```python
from build123d import *

# Parameters (mm, degrees)
SKETCH_W        = 50
SKETCH_H        = 50
PAD_DEPTH       = 10
SKETCH001_W     = 15
SKETCH001_H     = 50
PAD001_DEPTH    = 140
SKETCH004_R     = 2.6
POCKET002_DEPTH = 10
SKETCH005_R     = 8.5
SKETCH005_R_2   = 2.66237
SKETCH005_R_3   = 2.705532
POCKET_DEPTH    = 15
SKETCH006_W     = 50
SKETCH006_H     = 55
PAD002_DEPTH    = 50
SKETCH009_W     = 8
SKETCH009_H     = 50
PAD003_DEPTH    = 15
SKETCH010_R     = 8.5
POCKET003_DEPTH = 65
SKETCH011_R     = 18.1
POCKET004_DEPTH = 18
SKETCH012_R     = 2.570984
SKETCH012_R_2   = 2.587377
SKETCH012_R_3   = 2.575599
SKETCH012_R_4   = 2.613837
POCKET005_DEPTH = 65
CHAMFER_SIZE    = 7
CHAMFER001_SIZE = 7
SKETCH013_W     = 83.432911
SKETCH013_H     = 55
PAD004_DEPTH    = 4
SKETCH014_W     = 4
SKETCH014_H     = 55
PAD005_DEPTH    = 46
PAD006_DEPTH    = 4
PAD007_DEPTH    = 4
POCKET006_DEPTH = 5
SKETCH018_W     = 40
SKETCH018_H     = 35
PAD008_DEPTH    = 4
SKETCH019_R     = 1.6
POCKET007_DEPTH = 5
PAD009_DEPTH    = 3
PAD010_DEPTH    = 3
SKETCH022_R     = 2.1
POCKET008_DEPTH = 10
PAD011_DEPTH    = 50


with BuildPart() as part:
    # Sketch → Pad (new body)
    with BuildSketch(Plane.XY):
        with Locations((0, 25)):
            Rectangle(SKETCH_W, SKETCH_H)
    extrude(amount=PAD_DEPTH)

    # Sketch001 (on Face6 of Pad) → Pad001 (join)
    with BuildSketch(Plane.XY.offset(10)):
        with Locations((0, 25)):
            Rectangle(SKETCH001_W, SKETCH001_H)
    extrude(amount=PAD001_DEPTH)

    # Sketch004 → Pocket002 (cut)
    with BuildSketch(Plane(origin=(0, 0, 0), x_dir=(1, 0, 0), z_dir=(0, 0, -1))):
        with Locations((-20, -13)):
            Circle(SKETCH004_R)
        with Locations((20, -13)):
            Circle(SKETCH004_R)
        with Locations((-20, -37)):
            Circle(SKETCH004_R)
        with Locations((20, -37)):
            Circle(SKETCH004_R)
    extrude(amount=-POCKET002_DEPTH, mode=Mode.SUBTRACT)

    # Sketch005 (on Face14 of Pocket002) → Pocket (cut)
    with BuildSketch(Plane.YZ.offset(7.5)):
        with Locations((25, 50)):
            Circle(SKETCH005_R)
        with Locations((25, 120)):
            Circle(SKETCH005_R)
        with Locations((39.142136, 64.142136)):
            Circle(SKETCH005_R_2)
        with Locations((10.857864, 35.857864)):
            Circle(SKETCH005_R_3)
    extrude(amount=-POCKET_DEPTH, mode=Mode.SUBTRACT)

    # Sketch006 (on Face13 of Pocket) → Pad002 (join)
    with BuildSketch(Plane(origin=(-7.5, 0, 0), x_dir=(0, -1, 0), z_dir=(-1, 0, 0))):
        with Locations((-25, 122.5)):
            Rectangle(SKETCH006_W, SKETCH006_H)
    extrude(amount=PAD002_DEPTH)

    # Sketch009 → Pad003 (join)
    with BuildSketch(Plane.XY.offset(10)):
        with Locations((11.5, 25)):
            Rectangle(SKETCH009_W, SKETCH009_H)
        with Locations((-11.5, 25)):
            Rectangle(SKETCH009_W, SKETCH009_H)
    extrude(amount=PAD003_DEPTH)

    # Sketch010 (on Face34 of Pad003) → Pocket003 (cut)
    with BuildSketch(Plane.YZ.offset(-7.5)):
        with Locations((25, 120)):
            Circle(SKETCH010_R)
    extrude(amount=-POCKET003_DEPTH, mode=Mode.SUBTRACT)

    # Sketch011 (on DatumPlane) → Pocket004 (cut)
    with BuildSketch(Plane(origin=(-57.5, 0, 0), x_dir=(0, -1, 0), z_dir=(-1, 0, 0))):
        with Locations((-25, 120)):
            Circle(SKETCH011_R)
    extrude(amount=-POCKET004_DEPTH, mode=Mode.SUBTRACT)

    # Sketch012 (on DatumPlane) → Pocket005 (cut)
    with BuildSketch(Plane(origin=(-57.5, 0, 0), x_dir=(0, -1, 0), z_dir=(-1, 0, 0))):
        with Locations((-40.525694, 104.474306)):
            Circle(SKETCH012_R)
        with Locations((-40.524277, 135.524276)):
            Circle(SKETCH012_R_2)
        with Locations((-9.47356, 135.526441)):
            Circle(SKETCH012_R_3)
        with Locations((-9.442338, 104.444964)):
            Circle(SKETCH012_R_4)
    extrude(amount=-POCKET005_DEPTH, mode=Mode.SUBTRACT)

    # Chamfer
    chamfer_edges = [part.edges().sort_by_distance(p)[0] for p in [
        (15.5, 25, 25),
    ]]
    chamfer(chamfer_edges, length=CHAMFER_SIZE)

    # Chamfer001
    chamfer001_edges = [part.edges().sort_by_distance(p)[0] for p in [
        (-15.5, 25, 25),
    ]]
    chamfer(chamfer001_edges, length=CHAMFER001_SIZE)

    # Sketch013 (on DatumPlane) → Pad004 (join)
    with BuildSketch(Plane(origin=(0, 50, 0), x_dir=(-1, 0, 0), z_dir=(0, 1, 0))):
        with Locations((33.993362, 122.5)):
            Rectangle(SKETCH013_W, SKETCH013_H)
    extrude(amount=PAD004_DEPTH)

    # Sketch014 (on Face47 of Pad004) → Pad005 (join)
    with BuildSketch(Plane(origin=(0, 54, 0), x_dir=(-1, 0, 0), z_dir=(0, 1, 0))):
        with Locations((73.710442, 122.5)):
            Rectangle(SKETCH014_W, SKETCH014_H)
    extrude(amount=PAD005_DEPTH)

    # Sketch015 (on DatumPlane) → Pad006 (join)
    with BuildSketch(Plane.XY.offset(150)):
        Polygon((-71.717157, 54), (-11.717157, 54), (-71.717157, 87), align=None)
    extrude(amount=-PAD006_DEPTH)

    # Sketch016 (on DatumPlane) → Pad007 (join)
    with BuildSketch(Plane(origin=(0, 0, 95), x_dir=(1, 0, 0), z_dir=(0, 0, -1))):
        Polygon((-71.768631, -54), (-11.768631, -54), (-71.768631, -87), align=None)
    extrude(amount=-PAD007_DEPTH)

    # Sketch017 (on DatumPlane) → Pocket006 (cut)
    with BuildSketch(Plane(origin=(-75.710442, 0, 0), x_dir=(0, -1, 0), z_dir=(-1, 0, 0))):
        with BuildLine():
            ThreePointArc((-58.500315, 102.966849), (-56.900315, 104.566849), (-58.500315, 106.166849))
            Line((-58.500315, 106.166849), (-65.500315, 106.166849))
            ThreePointArc((-65.500315, 106.166849), (-67.100315, 104.566849), (-65.500315, 102.966849))
            Line((-65.500315, 102.966849), (-58.500315, 102.966849))
        make_face()
        with BuildLine():
            ThreePointArc((-89.5, 103.106524), (-87.9, 104.706524), (-89.5, 106.306524))
            Line((-89.5, 106.306524), (-96.5, 106.306524))
            ThreePointArc((-96.5, 106.306524), (-98.1, 104.706524), (-96.5, 103.106524))
            Line((-96.5, 103.106524), (-89.5, 103.106524))
        make_face()
        with BuildLine():
            ThreePointArc((-89.500832, 133.9), (-87.900832, 135.5), (-89.500832, 137.1))
            Line((-89.500832, 137.1), (-96.500832, 137.1))
            ThreePointArc((-96.500832, 137.1), (-98.100832, 135.5), (-96.500832, 133.9))
            Line((-96.500832, 133.9), (-89.500832, 133.9))
        make_face()
        with BuildLine():
            ThreePointArc((-58.500832, 133.9), (-56.900832, 135.5), (-58.500832, 137.1))
            Line((-58.500832, 137.1), (-65.500832, 137.1))
            ThreePointArc((-65.500832, 137.1), (-67.100832, 135.5), (-65.500832, 133.9))
            Line((-65.500832, 133.9), (-58.500832, 133.9))
        make_face()
        with BuildLine():
            ThreePointArc((-69.87661, 109), (-58.87661, 120), (-69.87661, 131))
            Line((-69.87661, 131), (-83.87661, 131))
            ThreePointArc((-83.87661, 131), (-94.87661, 120), (-83.87661, 109))
            Line((-83.87661, 109), (-69.87661, 109))
        make_face()
    extrude(amount=-POCKET006_DEPTH, mode=Mode.SUBTRACT)

    # Sketch018 (on DatumPlane) → Pad008 (join)
    with BuildSketch(Plane.XY.offset(150)):
        with Locations((-20, -17.5)):
            Rectangle(SKETCH018_W, SKETCH018_H)
    extrude(amount=-PAD008_DEPTH)

    # Sketch019 (on DatumPlane) → Pocket007 (cut)
    with BuildSketch(Plane.XY.offset(150)):
        with Locations((-10, -10)):
            Circle(SKETCH019_R)
        with Locations((-10, -25)):
            Circle(SKETCH019_R)
        with Locations((-35, -10)):
            Circle(SKETCH019_R)
        with Locations((-35, -25)):
            Circle(SKETCH019_R)
    extrude(amount=-POCKET007_DEPTH, mode=Mode.SUBTRACT)

    # Sketch020 (on DatumPlane) → Pad009 (join)
    with BuildSketch(Plane.YZ):
        Polygon((0, 146.040518), (-25, 146.040518), (0, 136.040518), align=None)
    extrude(amount=-PAD009_DEPTH)

    # Sketch021 (on DatumPlane) → Pad010 (join)
    with BuildSketch(Plane(origin=(-40, 0, 0), x_dir=(0, -1, 0), z_dir=(-1, 0, 0))):
        Polygon((0, 146), (25, 146), (0, 136), align=None)
    extrude(amount=-PAD010_DEPTH)

    # Sketch022 (on Face6 of Pocket006) → Pocket008 (cut)
    with BuildSketch(Plane.XZ):
        with Locations((0, 44.95862)):
            Circle(SKETCH022_R)
        with Locations((0, 64.95862)):
            Circle(SKETCH022_R)
    extrude(amount=-POCKET008_DEPTH, mode=Mode.SUBTRACT)

    # Sketch023 (on DatumPlane) → Pad011 (join)
    with BuildSketch(Plane.XZ):
        Polygon((-7.495659, 95), (-7.495659, 75), (-57.495659, 95), align=None)
    extrude(amount=-PAD011_DEPTH)


solid = part.part
```
The model under review builds one solid part; all positions refer to its coordinate system, in mm. A direction names the side the tool comes from. Coordinates: 2 decimals unless noted, no trailing zeros. Write each loop counter-clockwise with the first axis right and the second up, starting at its lowest first coordinate (ties: lowest second). Pieces come first, ordered by that corner, then holes. Notation, with made-up numbers: (-1.75, 68) -> (22.25, 68) arc R36 cw to (22.25, 103) -> close; hole circle Ø9 at (34.5, 38.25). An arc over 180 degrees is marked (long way). One line per item, written item: value. Start each with the question number.
Q1. Clearance check with flat-ended pins moving along their axes: P1, Ø1.3, axis at x = -0.5, z = 44.5, coming from the -Y side; P2, Ø6, axis at y = 24.5, z = 56.5, coming from the -X side; P3, Ø5, axis at x = 0, z = 44.96, coming from the -Y side. State where each tip first meets the part, or that it passes through.
Q2. Add section B-B, the plane x = 20. Give the boundary of the cut face in (y, z), then the cut area to 3 significant figures.
Q3. Add section A-A, the plane z = 120. Count the separate pieces of the cut face and the enclosed holes in it, then the cut area to 3 significant figures.
Q4. The part is to be moulded in two halves that separate along Y. For faces 4 (the face through (21.2, 15.307, 4.93)), 5 (the face through (-49, 65, 95)), 6 (the face through (0, 10, 65)), say which applies: +Y half, -Y half, draft (parallel to the pull), parting line (faces both ways), or undercut.
Q5. To check wall thickness, follow probe 1 along Y at (x, z) = (20, 2.25); probe 2 along Y at (x, z) = (-10, 148.3); probe 3 along Z at (x, y) = (-23, 26.5). State the ranges of each line that lie inside material, in increasing order.
Q6. For faces 1 (the face through (-20, 25, 10)), 2 (the face through (-0.27, 4.93, 67.04)), 3 (the face through (-17, 0, 91)), list the 3-axis set-ups (+Z, -Z, +X, -X, +Y, -Y) from which the entire face can be reached by the end or side of a thin tool; tool diameter is ignored.
Q7. Add section D-D, the plane y = 81. Give the boundary of the cut face in (x, z).
Response:
1. P1: y = 10
1. P2: x = -7.5
1. P3: y = 0
2. outline: (0, 0) -> (10.4, 0) -> (10.4, 10) -> (0, 10) -> close; (15.6, 0) -> (34.4, 0) -> (34.4, 10) -> (15.6, 10) -> close; (39.6, 0) -> (50, 0) -> (50, 10) -> (39.6, 10) -> close
2. area: 396 mm²
3. separate pieces: 3
3. enclosed holes: 0
3. area: 2,170 mm²
4. face 4: undercut
4. face 5: draft
4. face 6: -Y half
5. probe 1: 0 to 10.4, 15.6 to 34.4, 39.6 to 50
5. probe 2: -35 to -26.6, -23.4 to -11.6, -8.4 to 54
5. probe 3: 0 to 10, 81.2 to 111.63, 128.37 to 150
6. face 1: -X, +Y, -Y
6. face 2: -Y
6. face 3: -Z, -Y
7. outline: (-75.71, 95) -> (-60.86, 95) -> (-60.86, 99) -> (-71.71, 99) -> (-71.71, 109) -> (-75.71, 109) -> close; (-75.71, 131) -> (-71.71, 131) -> (-71.71, 146) -> (-60.81, 146) -> (-60.81, 150) -> (-75.71, 150) -> close
